For this review, take the finished solid that the model builds, in its own axes (mm). Round coordinates to 2 decimals unless told otherwise and drop trailing zeros. Order: outer loops, then holes, each group sorted by start corner. A loop starts at its lowest first (then second) coordinate and runs counter-clockwise, first axis right, second up. Notation, with made-up numbers: (68, 46.5) - (111, 46.5) arc R26 cw to (111, 63.5) - close; hole circle Ø7 at (-18, 77.25). An arc over 180 degrees is marked (long way). Write each question's results on one line, items separated by ' | '. Start each with the question number.
(1) Take a section at A-A, the plane y = 33. Give the boundary of the cut face in (x, z) (3 decimals), plus the area to 3 significant figures.
(2) For L1, parallel to X at y = -18, z = 0.25; L2, parallel to Z at x = 0, y = 5 (3 decimals); L3, parallel to Z at x = -1, y = 49, list the stretches that pass through material, from the lowest coordinate up. Write a range as from..to.
(3) Draft analysis for pull direction X (two halves, no side actions). For faces 1 (the flat face through (10, -1, 0)), 2 (the cylindrical face through (1.25, 1.38, -0.96)), 3 (the flat face through (2, 98.5, 0)), state which applies: pulls with the +X half, pulls with the -X half, needs draft (parallel to the pull), parting line crosses it, or undercut.
```python
from build123d import *

# Parameters (mm, degrees)
F0_W          = 20
F0_H          = 20
F1_DEPTH      = 98.5
F1_DEPTH_BACK = 98.5
F2_SIZE       = 5
F4_D          = 3.15


with BuildPart() as f1:
    # F0 (on Front) → F1 (new body, two sides)
    with BuildSketch(Plane.XZ) as f1_sk:
        Rectangle(F0_W, F0_H)
    extrude(amount=F1_DEPTH)
    extrude(f1_sk.sketch, amount=-F1_DEPTH_BACK)

    # F2
    f2_edges = [f1.edges().sort_by_distance(p)[0] for p in [
        (-10, 0, -10),
    ]]
    chamfer(f2_edges, length=F2_SIZE)

    # F4 (through all)
    with Locations(Plane.XZ.offset(98.5)):
        with Locations((0, 0)):
            Hole(F4_D / 2)


solid = f1.part
```
Results below:
1) outline: (-10, -5) - (-5, -10) - (10, -10) - (10, 10) - (-10, 10) - close; hole circle Ø3.15 at (0, 0) | area: 380 mm^2
2) L1: x = -10..-1.56, 1.56..10 | L2: z = -10..-1.575, 1.575..10 | L3: z = -10..-1.22, 1.22..10
3) face 1: pulls with the +X half | face 2: undercut | face 3: needs draft
